Input: dimensioned drawing with shaded views. Units: mm. Origin: part minimum x, y, z. A direction names the side the tool comes from. Give positions to 0.01 mm unless a question says otherwise; leave off trailing zeros. Write each loop counter-clockwise with the first axis right and the second up, starting at its lowest first coordinate (ties: lowest second). Pieces come first, ordered by that corner, then holes. Notation, with made-up numbers: (30.5, 13) -> (69.5, 13) arc R29 ccw to (69.5, 38) -> close; hole circle Ø9 at (39, -5.5). An arc over 180 degrees is marked (long way). Answer as a JSON object with one key per item and string values. Group by question number.
(1) Section query C-C on y = 13.75. Output: boundary loops of the cut face in (x, z), plus the area to 3 significant figures.
(2) Set-up query: the marked faces 1 and 2. Return all of +Z, -Z, +X, -X, +Y, -Y with unobstructed straight access to the full face (end or side cutting, diameter ignored); none if empty.
(3) Section query D-D on x = 40.5. Output: boundary loops of the cut face in (y, z).
(4) Contact query for flat-ended pins moving along their axis: pin 1 Ø1.1 at (x, z) = (30, 9) entering from -Y; pin 2 Ø0.7 at (y, z) = (20.5, 8.5) entering from -X; pin 3 Ø0.7 at (x, z) = (28.5, 9) entering from +Y. Output: stop coordinate, or through.
(5) Material intervals for probe 1 along Z at (x, y) = (38.5, 13); probe 2 along X at (y, z) = (14.5, 3); probe 3 along X at (y, z) = (8.5, 3.5) (1 decimal), sorted ascending.
(6) Section query B-B on y = 19.75. Output: boundary loops of the cut face in (x, z), plus the area to 3 significant figures.
(7) Section query A-A on z = 9.5. Output: boundary loops of the cut face in (x, y), plus the area to 3 significant figures.
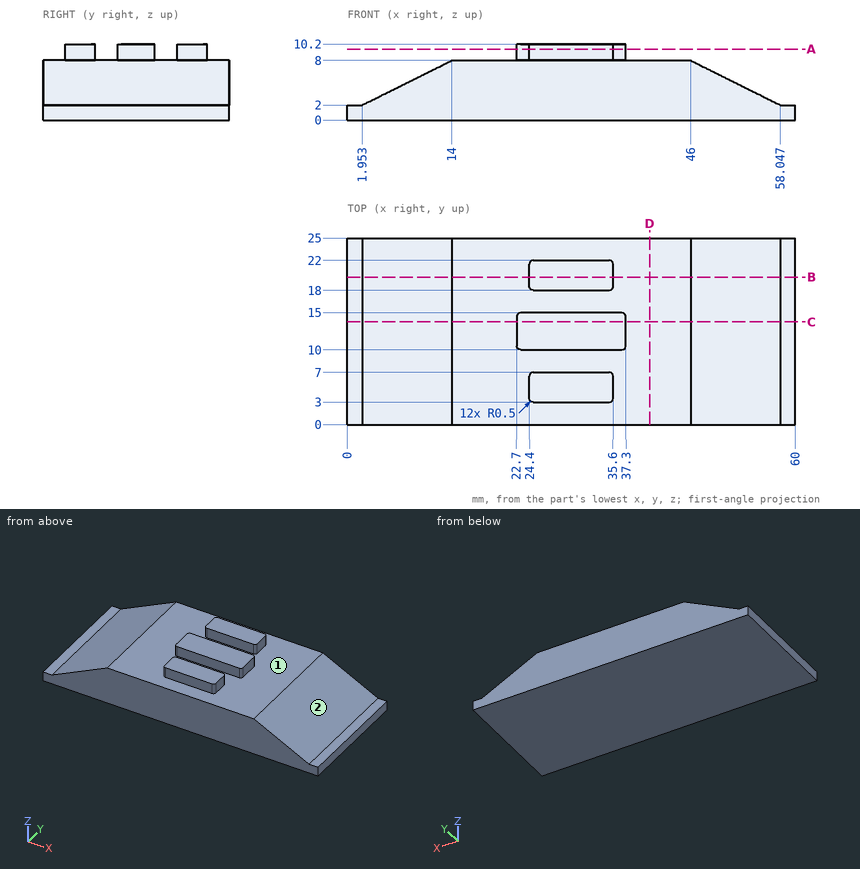
Answer list:
{
 "1": {"outline": "(0, 0) -> (60, 0) -> (60, 2) -> (58.05, 2) -> (46, 8) -> (37.3, 8) -> (37.3, 10.2) -> (22.7, 10.2) -> (22.7, 8) -> (14, 8) -> (1.95, 2) -> (0, 2) -> close", "area": "416 mm2"},
 "2": {"face 1": "+Z", "face 2": "+Z, +X, +Y, -Y"},
 "3": {"outline": "(0, 0) -> (25, 0) -> (25, 8) -> (0, 8) -> close"},
 "4": {"pin 1": "y = 3", "pin 2": "x = 24.4", "pin 3": "y = 22"},
 "5": {"probe 1": "0 to 8", "probe 2": "3.96 to 56.04", "probe 3": "5 to 55"},
 "6": {"outline": "(0, 0) -> (60, 0) -> (60, 2) -> (58.05, 2) -> (46, 8) -> (35.6, 8) -> (35.6, 10.2) -> (24.4, 10.2) -> (24.4, 8) -> (14, 8) -> (1.95, 2) -> (0, 2) -> close", "area": "409 mm2"},
 "7": {"outline": "(22.7, 10.5) arc R0.5 ccw to (23.2, 10) -> (36.8, 10) arc R0.5 ccw to (37.3, 10.5) -> (37.3, 14.5) arc R0.5 ccw to (36.8, 15) -> (23.2, 15) arc R0.5 ccw to (22.7, 14.5) -> close; (24.4, 3.5) arc R0.5 ccw to (24.9, 3) -> (35.1, 3) arc R0.5 ccw to (35.6, 3.5) -> (35.6, 6.5) arc R0.5 ccw to (35.1, 7) -> (24.9, 7) arc R0.5 ccw to (24.4, 6.5) -> close; (24.4, 18.5) arc R0.5 ccw to (24.9, 18) -> (35.1, 18) arc R0.5 ccw to (35.6, 18.5) -> (35.6, 21.5) arc R0.5 ccw to (35.1, 22) -> (24.9, 22) arc R0.5 ccw to (24.4, 21.5) -> close", "area": "162 mm2"}
}
